```python
from build123d import *

# Parameters (mm, degrees)
SKETCH1_R           = 6
BOSS_EXTRUDE1_DEPTH = 50
SKETCH2_R           = 10
BOSS_EXTRUDE2_DEPTH = 5
SKETCH3_W           = 7
SKETCH3_H           = 7
BOSS_EXTRUDE3_DEPTH = 10


with BuildPart() as part:
    # Sketch1 → Boss-Extrude1 (new body)
    with BuildSketch(Plane.XY):
        Circle(SKETCH1_R)
    extrude(amount=BOSS_EXTRUDE1_DEPTH)

    # Sketch2 → Boss-Extrude2 (add)
    with BuildSketch(Plane(origin=(0, 0, 0), x_dir=(-1, 0, 0), z_dir=(0, 0, -1))):
        Circle(SKETCH2_R)
    extrude(amount=-BOSS_EXTRUDE2_DEPTH)

    # Sketch3 → Boss-Extrude3 (add)
    with BuildSketch(Plane.XY.offset(50)):
        Rectangle(SKETCH3_W, SKETCH3_H)
    extrude(amount=BOSS_EXTRUDE3_DEPTH)


solid = part.part
```
Here's how the part is built. I have some questions about the finished solid (model axes, mm). A direction names the side the tool comes from. Round coordinates to 2 decimals unless told otherwise and drop trailing zeros. Order: outer loops, then holes, each group sorted by start corner. A loop starts at its lowest first (then second) coordinate and runs counter-clockwise, first axis right, second up. Notation, with made-up numbers: (84, 88) -> (120, 88) arc R25 ccw to (120, 116) -> close; hole circle Ø5 at (75.25, -10). An arc over 180 degrees is marked (long way). Use a Markdown table: item, result. Add a question column.
(1) I need wall thicknesses on line 1 along X through (y, z) = (0.25, 33.5); line 2 along Y through (x, z) = (0, 57.5); line 3 along Z through (x, y) = (1.25, -8.75). Which ranges of each line are inside material? Lowest first, please.
(2) Suppose I cut it at D-D, the plane y = 5.25. Please give me the cut outline in (x, z), and give its area (3 significant figures).
(3) Suppose I cut it at A-A, the plane x = 0. Please give me the cut outline in (y, z).
(4) Suppose I cut it at C-C, the plane z = 40. Please give me the cut outline in (x, y).
(5) For faces 1 (the face through (0, 3.5, 55)), 2 (the face through (-3.5, 0, 55)), 3 (the face through (-6, 0, 27)), 4 (the face through (3.5, 0, 55)), which set-ups out of +Z, -Z, +X, -X, +Y, -Y let a thin tool reach every point of the face, with its end or its side?
(6) For pin 1 Ø3.5 at (y, z) = (0, 54) entering from +X; pin 2 Ø10 at (y, z) = (5.5, 26.5) entering from +X; pin 3 Ø5 at (x, z) = (4, 13) entering from -Y; pin 4 Ø1 at (x, z) = (7.5, 21.5) entering from +Y, each with a flat end and sliding along its axis, tell me the tip position at first contact or that it passes through.
Verdict:
| question | item | result |
|---|---|---|
| 1 | line 1 | -5.99 to 5.99 |
| 1 | line 2 | -3.5 to 3.5 |
| 1 | line 3 | 0 to 5 |
| 2 | outline | (-8.51, 0) -> (8.51, 0) -> (8.51, 5) -> (2.9, 5) -> (2.9, 50) -> (-2.9, 50) -> (-2.9, 5) -> (-8.51, 5) -> close |
| 2 | area | 347 mm2 |
| 3 | outline | (-10, 0) -> (10, 0) -> (10, 5) -> (6, 5) -> (6, 50) -> (3.5, 50) -> (3.5, 60) -> (-3.5, 60) -> (-3.5, 50) -> (-6, 50) -> (-6, 5) -> (-10, 5) -> close |
| 4 | outline | circle Ø12 at (0, 0) |
| 5 | face 1 | +Z, +X, -X, +Y |
| 5 | face 2 | +Z, -X, +Y, -Y |
| 5 | face 3 | +Z |
| 5 | face 4 | +Z, +X, +Y, -Y |
| 6 | pin 1 | x = 3.5 |
| 6 | pin 2 | x = 5.98 |
| 6 | pin 3 | y = -5.81 |
| 6 | pin 4 | through |
